Read the model definition and answer for the solid it produces. Units are mm, in the model's axes. A direction names the side the tool comes from. Coordinates: 2 decimals unless noted, no trailing zeros. Write each loop counter-clockwise with the first axis right and the second up, starting at its lowest first coordinate (ties: lowest second). Pieces come first, ordered by that corner, then holes. Notation, with made-up numbers: (54.25, 52.25) -> (112.25, 52.25) arc R17 ccw to (112.25, 58.25) -> close; hole circle Ø7 at (13.25, 48). An arc over 180 degrees is marked (long way). Answer in a Markdown table with one row per item. Add a question column.
Item 1: Given pin 1 Ø1.1 at (x, z) = (61, 17.5) entering from -Y; pin 2 Ø1 at (x, z) = (61.5, 10) entering from -Y; pin 3 Ø1.5 at (y, z) = (57.5, 14) entering from +X; pin 4 Ø4 at (x, y) = (44.5, 11.5) entering from -Z, each flat-ended and moving along its own axis, determine where each tip first touches the part or whether it passes through.
Item 2: Section D-D on y = 74 is taken. Write down the section's boundary in (x, z), then the cut area to 3 significant figures.
Item 3: Straight lines are drawn through the part: line 1 (Y direction, x = 52, z = 14.75); line 2 (X direction, y = 47, z = 29); line 3 (X direction, y = 29, z = 22.5). For each, find the intervals that lie inside material, in ascending order. Write a range as from..to.
Item 4: Section B-B on z = 22.75 is taken. Write down the section's boundary in (x, y), then the cut area to 3 significant figures.
Item 5: For a pull along Y with two mould halves and no side action, classify faces 1 (the face through (62, 5, 13)), 2 (the face through (64, 32, 4)), 3 (the face through (29, 88, 14)) as +Y half, -Y half, draft (parallel to the pull), parting line (faces both ways), or undercut.
Item 6: Section A-A on y = 47 is taken. Write down the section's boundary in (x, z), then the cut area to 3 significant figures.
Item 7: Section C-C on x = 35 is taken. Write down the section's boundary in (y, z), then the cut area to 3 significant figures.
Item 8: Which of the six approach directions +Z, -Z, +X, -X, +Y, -Y give full straight-line access (tool end or side, diameter ignored) to faces 4 (the face through (60.5, 50, 22)), 5 (the face through (62, 41, 21)), 6 (the face through (62, 11, 21))?
```python
from build123d import *

# Parameters (mm, degrees)
F0_W      = 59
F0_H      = 83
F0_W_2    = 43
F0_H_2    = 67
F1_DEPTH  = 3
F2_R      = 1.45
F3_DEPTH  = 7
F4_W      = 69
F4_H      = 93
F4_W_2    = 59
F4_H_2    = 83
F5_DEPTH  = 28
F6_R      = 2.45
F7_DEPTH  = 2
F9_DEPTH  = 5
F10_W     = 15
F10_H     = 20
F10_W_2   = 3
F10_H_2   = 15
F11_DEPTH = 5
F12_W     = 62
F12_H     = 86
F12_R     = 2.5
F13_DEPTH = 25
F15_W     = 10
F15_H     = 3
F16_DEPTH = 3.5
F17_W     = 25
F17_H     = 20
F18_DEPTH = 2.5
F21_DEPTH = 76
F23_W     = 1.5
F23_H     = 2
F24_DEPTH = 52
F25_R     = 4.99999


# Not quite as in the source:
# - a fillet or chamfer is up to 0.001 mm smaller than in the source, because OpenCascade refuses the exact size


with BuildPart() as f1:
    # F0 (on Top) → F1 (new body)
    with BuildSketch(Plane.XY):
        with Locations((29.5, 41.5)):
            Rectangle(F0_W, F0_H)
        with Locations((29.5, 41.5)):
            Rectangle(F0_W_2, F0_H_2, mode=Mode.SUBTRACT)
    extrude(amount=F1_DEPTH)

    # F2 (on face) → F3 (join)
    with BuildSketch(Plane.XY.offset(3)):
        with Locations((3.5, 3.5)):
            Circle(F2_R)
        with Locations((55.5, 3.5)):
            Circle(F2_R)
        with Locations((3.5, 79.5)):
            Circle(F2_R)
        with Locations((55.5, 79.5)):
            Circle(F2_R)
    extrude(amount=F3_DEPTH)

    # F4 (on Top) → F5 (join)
    with BuildSketch(Plane.XY):
        with Locations((29.5, 41.5)):
            Rectangle(F4_W, F4_H)
        with Locations((29.5, 41.5)):
            Rectangle(F4_W_2, F4_H_2, mode=Mode.SUBTRACT)
    extrude(amount=F5_DEPTH)

    # F6 (on face) → F7 (join)
    with BuildSketch(Plane.XY.offset(3)):
        with Locations((3.5, 79.5)):
            Circle(F6_R)
        with Locations((55.5, 79.5)):
            Circle(F6_R)
        with Locations((55.5, 3.5)):
            Circle(F6_R)
        with Locations((3.5, 3.5)):
            Circle(F6_R)
    extrude(amount=F7_DEPTH)

    # F8 (on face) → F9 (cut, through all)
    with BuildSketch(Plane(origin=(-5, 0, 0), x_dir=(0, -1, 0), z_dir=(-1, 0, 0))):
        Polygon((-79, 20), (-79, 5), (-77, 5), (-77, 3), (-37, 3), (-37, 5), (-4, 5), (-4, 20), (-37, 20), (-37, 25), (-77, 25), (-77, 20), align=None)
    extrude(amount=-F9_DEPTH, mode=Mode.SUBTRACT)

    # F10 (on face) → F11 (cut, through all)
    with BuildSketch(Plane.YZ.offset(64)):
        with Locations((67.85, 15)):
            Rectangle(F10_W, F10_H)
        with Locations((1.5, 13.5)):
            Rectangle(F10_W_2, F10_H_2)
        with Locations((6.5, 13.5)):
            Rectangle(F10_W_2, F10_H_2)
        with Locations((11.5, 13.5)):
            Rectangle(F10_W_2, F10_H_2)
        with Locations((16.5, 13.5)):
            Rectangle(F10_W_2, F10_H_2)
        with Locations((21.5, 13.5)):
            Rectangle(F10_W_2, F10_H_2)
        with Locations((26.5, 13.5)):
            Rectangle(F10_W_2, F10_H_2)
        with Locations((31.5, 13.5)):
            Rectangle(F10_W_2, F10_H_2)
        with Locations((36.5, 13.5)):
            Rectangle(F10_W_2, F10_H_2)
        with Locations((41.5, 13.5)):
            Rectangle(F10_W_2, F10_H_2)
        with Locations((46.5, 13.5)):
            Rectangle(F10_W_2, F10_H_2)
        with Locations((51.5, 13.5)):
            Rectangle(F10_W_2, F10_H_2)
    extrude(amount=-F11_DEPTH, mode=Mode.SUBTRACT)

    # F12 (on face) → F13 (cut)
    with BuildSketch(Plane.XY.offset(3)):
        with Locations((29.5, 41.5)):
            Rectangle(F12_W, F12_H)
        with Locations((3.5, 3.5)):
            Circle(F12_R, mode=Mode.SUBTRACT)
        with Locations((55.5, 3.5)):
            Circle(F12_R, mode=Mode.SUBTRACT)
        with Locations((3.5, 79.5)):
            Circle(F12_R, mode=Mode.SUBTRACT)
        with Locations((55.5, 79.5)):
            Circle(F12_R, mode=Mode.SUBTRACT)
    extrude(amount=F13_DEPTH, mode=Mode.SUBTRACT)

    # F15 (on face) → F16 (cut)
    with BuildSketch(Plane(origin=(-5, 0, 0), x_dir=(0, -1, 0), z_dir=(-1, 0, 0))):
        with Locations((-54.22, 1.5)):
            Rectangle(F15_W, F15_H)
    extrude(amount=-F16_DEPTH, mode=Mode.SUBTRACT)

    # F17 (on face) → F18 (cut)
    with BuildSketch(Plane.YZ.offset(64)):
        with Locations((67.85, 15)):
            Rectangle(F17_W, F17_H)
    extrude(amount=-F18_DEPTH, mode=Mode.SUBTRACT)

    # F20 (on offset) → F21 (join)
    with BuildSketch(Plane.XZ.offset(-79.5)):
        with BuildLine():
            Line((-2.5, 29), (-2.5, 28))
            Line((-2.5, 28), (-1.5, 28))
            Line((-1.5, 28), (-1.5, 30))
            Line((-1.5, 30), (-3, 30))
            ThreePointArc((-3, 30), (-2.8716037917, 29.4391981041), (-2.5, 29))
        make_face()
        with BuildLine():
            Line((60.5, 28), (61.5, 28))
            Line((61.5, 28), (61.5, 29))
            ThreePointArc((61.5, 29), (61.8716037917, 29.4391981041), (62, 30))
            Line((62, 30), (60.5, 30))
            Line((60.5, 30), (60.5, 28))
        make_face()
    extrude(amount=F21_DEPTH)

    # F23 (on offset) → F24 (join)
    with BuildSketch(Plane.YZ.offset(3.5)):
        with Locations((-2.25, 29)):
            Rectangle(F23_W, F23_H)
        with Locations((85.25, 29)):
            Rectangle(F23_W, F23_H)
    extrude(amount=F24_DEPTH)

    # F25 (radius 5 in the source; OpenCascade refuses exactly that, so slightly less here)
    f25_edges = [f1.edges().sort_by_distance(p)[0] for p in [
        (-5, -5, 14),
        (64, -5, 14),
        (64, 88, 14),
        (-5, 88, 14),
    ]]
    fillet(f25_edges, radius=F25_R)


solid = f1.part
```
Results below:
| question | item | result |
|---|---|---|
| 1 | pin 1 | stops at y = -4.79 |
| 1 | pin 2 | stops at y = -4.58 |
| 1 | pin 3 | stops at x = 61.5 |
| 1 | pin 4 | passes through |
| 2 | outline | (-5, 0) -> (8, 0) -> (8, 3) -> (-5, 3) -> close; (-5, 25) -> (-1.5, 25) -> (-1.5, 30) -> (-3, 30) arc R1.22 ccw to (-2.5, 29) -> (-2.5, 28) -> (-5, 28) -> close; (51, 0) -> (64, 0) -> (64, 5) -> (60.5, 5) -> (60.5, 3) -> (51, 3) -> close; (60.5, 25) -> (64, 25) -> (64, 28) -> (61.5, 28) -> (61.5, 29) arc R1.22 ccw to (62, 30) -> (60.5, 30) -> close |
| 2 | area | 111 mm2 |
| 3 | line 1 | y = -5..-1.5, 84.5..88 |
| 3 | line 2 | x = -2.5..-1.5, 60.5..61.5 |
| 3 | line 3 | x = -5..-1.5, 60.5..64 |
| 4 | outline | (-5, 0) arc R5 ccw to (0, -5) -> (59, -5) arc R5 ccw to (64, 0) -> (64, 55.35) -> (61.5, 55.35) -> (61.5, 60.35) -> (60.5, 60.35) -> (60.5, -1.5) -> (-1.5, -1.5) -> (-1.5, 37) -> (-5, 37) -> close; (-5, 77) -> (-1.5, 77) -> (-1.5, 84.5) -> (60.5, 84.5) -> (60.5, 75.35) -> (61.5, 75.35) -> (61.5, 80.35) -> (64, 80.35) -> (64, 83) arc R5 ccw to (59, 88) -> (0, 88) arc R5 ccw to (-5, 83) -> close |
| 4 | area | 846 mm2 |
| 5 | face 1 | undercut |
| 5 | face 2 | draft |
| 5 | face 3 | +Y half |
| 6 | outline | (-5, 0) -> (8, 0) -> (8, 3) -> (-5, 3) -> close; (-5, 25) -> (-1.5, 25) -> (-1.5, 30) -> (-3, 30) arc R1.22 ccw to (-2.5, 29) -> (-2.5, 28) -> (-5, 28) -> close; (51, 0) -> (64, 0) -> (64, 6) -> (60.5, 6) -> (60.5, 3) -> (51, 3) -> close; (60.5, 21) -> (64, 21) -> (64, 28) -> (61.5, 28) -> (61.5, 29) arc R1.22 ccw to (62, 30) -> (60.5, 30) -> close |
| 6 | area | 128 mm2 |
| 7 | outline | (-5, 0) -> (8, 0) -> (8, 3) -> (-1.5, 3) -> (-1.5, 30) -> (-3, 30) -> (-3, 28) -> (-5, 28) -> close; (75, 0) -> (88, 0) -> (88, 28) -> (86, 28) -> (86, 30) -> (84.5, 30) -> (84.5, 3) -> (75, 3) -> close |
| 7 | area | 259 mm2 |
| 8 | face 4 | +Z |
| 8 | face 5 | +X, -X |
| 8 | face 6 | +X |
